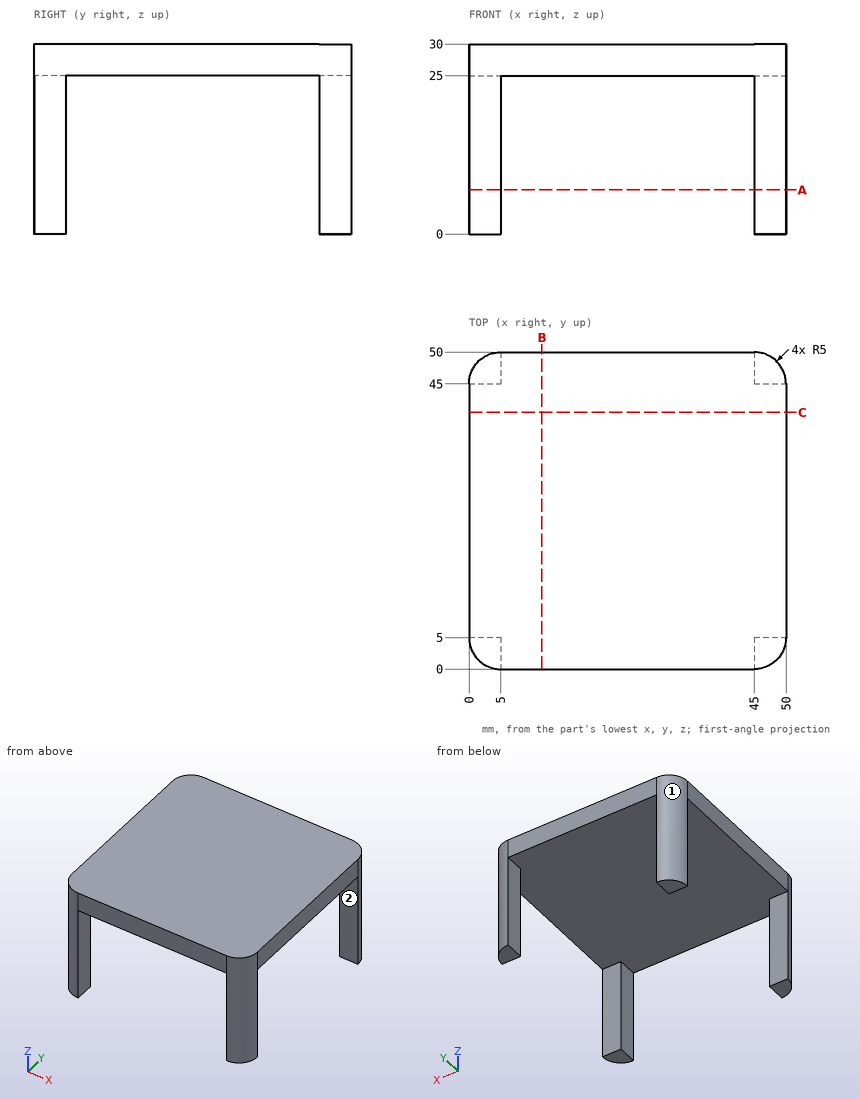
Check sheet for the drawn part. Datum: minimum x, y, z corner. Units: mm. A direction names the side the tool comes from. Give positions to 0.01 mm unless a question says otherwise; leave off trailing zeros. Loops run counter-clockwise (first coordinate to the right, second up) from the corner with the lowest first, then second, coordinate; pieces in that order, holes last. Notation, with made-up numbers: M -9.75,6 L 48.25,6 A34 cw 48.25,42 Z; hole C 17,74.5 d1. An arc over 180 degrees is marked long. Answer as CSV lines item,"result".
Item 1: Scan lines: L1, parallel to Z at x = 38.5, y = 13; L2, parallel to Y at x = 47, z = 3.25; L3, parallel to X at y = 46.5, z = 1.75. Record each from-to range of solid material in increasing order.
Reply:
L1,"25 to 30"
L2,"0.42 to 5, 45 to 49.58"
L3,"0.23 to 5, 45 to 49.77"
Item 2: Depth check by flat-ended pin: pin 1 Ø3 at (x, y) = (41, 40) entering from -Z; pin 2 Ø5.5 at (y, z) = (47, 7.5) entering from +X; pin 3 Ø4 at (y, z) = (2, 15) entering from +X; pin 4 Ø1.5 at (y, z) = (47, 9) entering from -X. Enter the tip coordinate at first touch or a pass-through.
Reply:
pin 1,"z = 25"
pin 2,"x = 50"
pin 3,"x = 49.9"
pin 4,"x = 0.16"
Item 3: Sectioned sample at A-A, the plane z = 7. State how many separate pieces and enclosed holes the cut face has, then the cut area to 3 significant figures.
Reply:
separate pieces,"4"
enclosed holes,"0"
area,"78.5 mm^2"
Item 4: Set-up check for the marked faces 1 and 2: record each of +Z, -Z, +X, -X, +Y, -Y from which the full face is reachable in a straight line by a thin tool's end or side.
Reply:
face 1,"+Z, -Z, -X, +Y"
face 2,"-Z, +X, -X"
Item 5: Sectioned sample at B-B, the plane x = 11.5. Enter the section's corners in (y, z), then the cut area to 3 significant figures.
Reply:
outline,"M 0,25 L 50,25 L 50,30 L 0,30 Z"
area,"250 mm^2"
